Geometry: see drawing. Coordinates: mm, zero at the bounding-box minimum. A direction names the side the tool comes from. Round coordinates to 2 decimals unless told otherwise and drop trailing zeros. Write each loop counter-clockwise with the first axis right and the second up, starting at its lowest first coordinate (ties: lowest second). Pieces come first, ordered by that corner, then holes. Notation, with made-up numbers: (78, 39.25) - (108, 39.25) arc R17 cw to (108, 56.25) - close; hole circle Ø10 at (85, 30). An arc over 180 degrees is marked (long way). One line per item, written item: value. Start each with the question number.
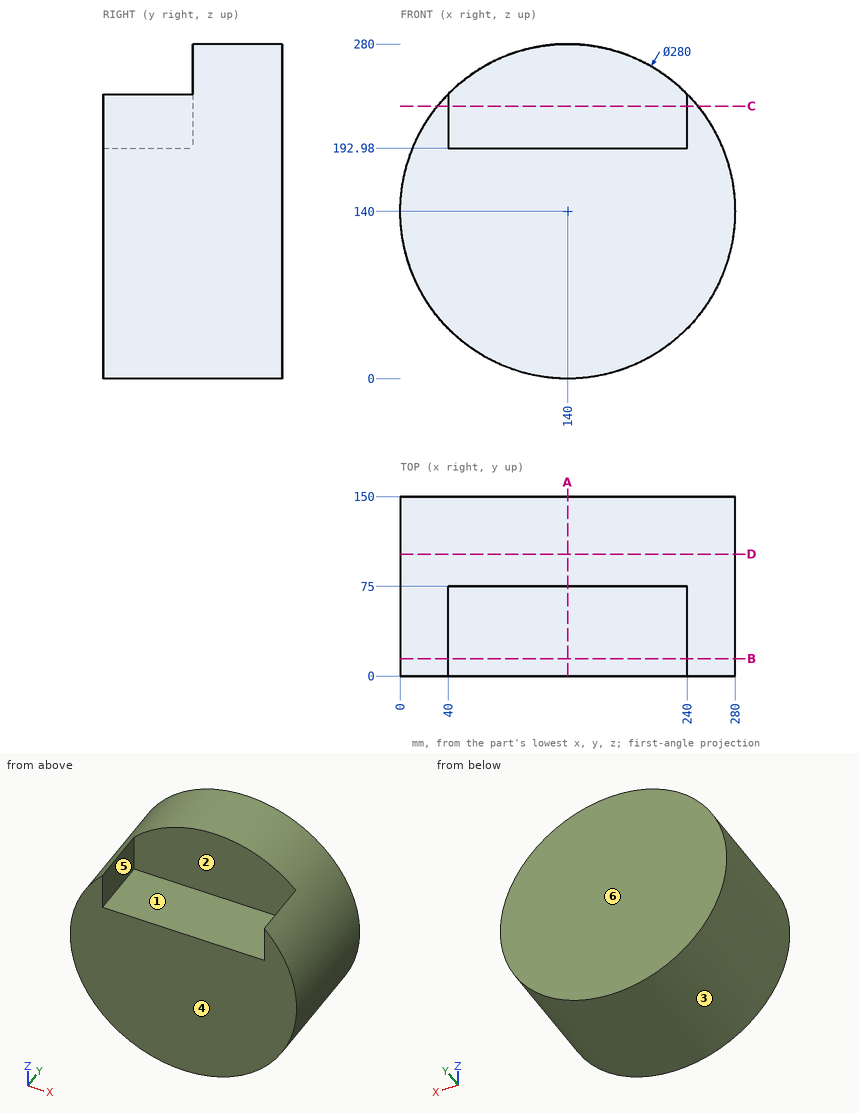
Q1. Pull-direction query (X, two-part tool) for the marked faces 1, 2, 3 and 4; classes: pulls with the +X half, pulls with the -X half, needs draft (parallel to the pull), parting line crosses it, or undercut.
Q2. Cut plane D-D, the plane y = 102. Output: boundary loops of the cut face in (x, z).
Q3. Contact query for flat-ended pins moving along their axis: pin 1 Ø1 at (y, z) = (32, 195.5) entering from -X; pin 2 Ø22.5 at (y, z) = (27.5, 211) entering from -X; pin 3 Ø3 at (x, y) = (242.5, 88.5) entering from -Z. Output: stop coordinate, or through.
Q4. Cut plane A-A, the plane x = 140. Output: boundary loops of the cut face in (y, z), and give its area (3 significant figures).
Q5. Cut plane B-B, the plane y = 14.5. Output: boundary loops of the cut face in (x, z).
Q6. Material intervals for probe 1 along Y at (x, z) = (196, 229); probe 2 along X at (y, z) = (64.5, 228.5); probe 3 along Z at (x, y) = (191.5, 17) (1 decimal), sorted ascending. Write a range as from..to.
Q7. Access query for the marked faces 5 and 6. Directions: +Z, -Z, +X, -X, +Y, -Y. A direction counts if a zero-diameter tool reaches every point of the face in a straight line with its end or side. Return the directions, or none.
Q8. Cut plane C-C, the plane z = 228. Output: boundary loops of the cut face in (x, y) (1 decimal), and give its area (3 significant figures).
A:
1. face 1: undercut
1. face 2: undercut
1. face 3: parting line crosses it
1. face 4: needs draft
2. outline: circle Ø280 at (140, 140)
3. pin 1: stops at x = 11.26
3. pin 2: stops at x = 13.39
3. pin 3: stops at z = 43.05
4. outline: (0, 0) - (150, 0) - (150, 280) - (75, 280) - (75, 192.98) - (0, 192.98) - close
4. area: 35,500 mm²
5. outline: (40, 192.98) - (40, 237.98) arc R140 ccw (long way) to (240, 237.98) - (240, 192.98) - close
6. probe 1: y = 75..150
6. probe 2: x = 31.52..40, 240..248.48
6. probe 3: z = 9.8..193
7. face 5: +Z, -Y
7. face 6: +Z, -Z, +X, -X, +Y
8. outline: (31.1, 0) - (40, 0) - (40, 75) - (240, 75) - (240, 0) - (248.9, 0) - (248.9, 150) - (31.1, 150) - close
8. area: 17,700 mm²
